Verification items for the finished model (mm, model axes). A direction names the side the tool comes from. Round coordinates to 2 decimals unless told otherwise and drop trailing zeros. Order: outer loops, then holes, each group sorted by start corner. A loop starts at its lowest first (then second) coordinate and runs counter-clockwise, first axis right, second up. Notation, with made-up numbers: (34.25, 31) -> (47.25, 31) arc R5 ccw to (47.25, 36) -> close; hole circle Ø4 at (31, 1). An arc over 180 degrees is marked (long way). Put each result on its own line as item: value.
```python
from build123d import *

# Parameters (mm, degrees)
F1_DEPTH       = 27.5
F0_R           = 8
F2_DEPTH       = 9.5
F5_D           = 3
F5_CSINK_D     = 8
F5_CSINK_ANGLE = 90
F6_W           = 26
F6_H           = 50
F6_R           = 1.5
F7_DEPTH       = 5


with BuildPart() as f1:
    # F0 (on Front) → F1 (new body, symmetric)
    with BuildSketch(Plane.XZ):
        Polygon((-15, 4.5), (-15, -4.5), (15, -4.5), (15, 0.0487750938), (15, 4.5), align=None)
    extrude(amount=F1_DEPTH, both=True)

    # F0 (on Front) → F2 (join, symmetric)
    with BuildSketch(Plane.XZ):
        with BuildLine():
            Line((15, 4.5), (15, 0.0487750938))
            Line((15, 0.0487750938), (26.0270317086, 0.0487750938))
            ThreePointArc((26.0270317086, 0.0487750938), (20.4485510909, 1.7874477446), (16.5475113082, 6.1376566135))
            ThreePointArc((16.5475113082, 6.1376566135), (16.1265778305, 4.9854273341), (15, 4.5))
        make_face()
        with BuildLine():
            ThreePointArc((16.5475113082, 6.1376566135), (20.4485510909, 1.7874477446), (26.0270317086, 0.0487750938))
            ThreePointArc((26.0270317086, 0.0487750938), (34.040923726, 3.1360416589), (37.393363731, 11.0426734401))
            ThreePointArc((37.393363731, 11.0426734401), (24.4033695136, 21.8611725511), (16.1133777283, 7.1283551362))
            ThreePointArc((16.1133777283, 7.1283551362), (16.4196666887, 6.6721038843), (16.5475113082, 6.1376566135))
        make_face()
        with Locations((26.393363731, 11.0426734401)):
            Circle(F0_R, mode=Mode.SUBTRACT)
    extrude(amount=F2_DEPTH, both=True)

    # F5 (through all)
    with Locations(Plane.XY.offset(4.5)):
        with Locations((3, 18.5), (3, -18.5)):
            CounterSinkHole(F5_D / 2, F5_CSINK_D / 2, counter_sink_angle=F5_CSINK_ANGLE)

    # F6 (on face) → F7 (cut)
    with BuildSketch(Plane(origin=(0, 0, -4.5), x_dir=(1, 0, 0), z_dir=(0, 0, -1))):
        Rectangle(F6_W, F6_H)
        with Locations((3, -18.5)):
            Circle(F6_R, mode=Mode.SUBTRACT)
        with Locations((3, 18.5)):
            Circle(F6_R, mode=Mode.SUBTRACT)
    extrude(amount=-F7_DEPTH, mode=Mode.SUBTRACT)


solid = f1.part
```
Item 1: Release check for a two-part mould opening along Z. For faces 1 (the face through (0, 0, 0.5)), 2 (the face through (3, -17, 1)), 3 (the face through (3.35, -20.08, 2.12)), 4 (the face through (18.4, 0.1, 11.4)) record: pulls with the +Z half, pulls with the -Z half, needs draft (parallel to the pull), parting line crosses it, or undercut.
Geometry check:
face 1: pulls with the -Z half
face 2: needs draft
face 3: pulls with the +Z half
face 4: undercut
Item 2: Material ranges on line 1 along Y through (x, z) = (3, 1.6); line 2 along X through (y, z) = (18.5, 1.3); line 3 along Y through (x, z) = (3, 0), recorded low to high.
Geometry check:
line 1: -27.5 to -20, -17 to 17, 20 to 27.5
line 2: -15 to 1.5, 4.5 to 15
line 3: -27.5 to -25, 25 to 27.5
Item 3: Depth check by flat-ended pin: pin 1 Ø1.5 at (y, z) = (9, -1) entering from +X; pin 2 Ø1.5 at (y, z) = (-7, 5.5) entering from +X; pin 3 Ø4 at (x, y) = (3, -18.5) entering from -Z; pin 4 Ø13 at (x, z) = (26.39, 11.04) entering from +Y. Enter the tip coordinate at first touch or a pass-through.
Geometry check:
pin 1: x = 15
pin 2: x = 36.29
pin 3: z = 0.5
pin 4: through
Item 4: Tool access check on faces 5 (the face through (0, 0, 4.5)), 6 (the face through (0, -25, -2)), 7 (the face through (20, 0, 0.049)), 8 (the face through (18.6, -9.5, 13.6)), 9 (the face through (18.6, 9.5, 13.6)). Record the directions out of +Z, -Z, +X, -X, +Y, -Y that give a thin tool (end or side, any length) a straight path to the whole face; none if there is none.
Geometry check:
face 5: +Z, -X, +Y, -Y
face 6: -Z
face 7: -Z, +X, +Y, -Y
face 8: +Z, -Z, +X, -Y
face 9: +Z, -Z, +X, +Y
Item 5: Sectioned sample at A-A, the plane y = 18.5. Record the boundary of the cut face in (x, z).
Geometry check:
outline: (-15, -4.5) -> (-13, -4.5) -> (-13, 0.5) -> (1.5, 0.5) -> (1.5, 2) -> (-1, 4.5) -> (-15, 4.5) -> close; (4.5, 0.5) -> (13, 0.5) -> (13, -4.5) -> (15, -4.5) -> (15, 4.5) -> (7, 4.5) -> (4.5, 2) -> close
Item 6: Sectioned sample at B-B, the plane x = 3. Record the boundary of the cut face in (y, z).
Geometry check:
outline: (-27.5, -4.5) -> (-25, -4.5) -> (-25, 0.5) -> (-20, 0.5) -> (-20, 2) -> (-22.5, 4.5) -> (-27.5, 4.5) -> close; (-17, 0.5) -> (17, 0.5) -> (17, 2) -> (14.5, 4.5) -> (-14.5, 4.5) -> (-17, 2) -> close; (20, 0.5) -> (25, 0.5) -> (25, -4.5) -> (27.5, -4.5) -> (27.5, 4.5) -> (22.5, 4.5) -> (20, 2) -> close
Item 7: Sectioned sample at D-D, the plane z = 16.5. Record the boundary of the cut face in (x, y), then the cut area to 3 significant figures.
Geometry check:
outline: (16.84, -9.5) -> (20.54, -9.5) -> (20.54, 9.5) -> (16.84, 9.5) -> close; (32.24, -9.5) -> (35.94, -9.5) -> (35.94, 9.5) -> (32.24, 9.5) -> close
area: 141 mm2
Item 8: Sectioned sample at C-C, the plane x = 29. Record the boundary of the cut face in (y, z).
Geometry check:
outline: (-9.5, 0.36) -> (9.5, 0.36) -> (9.5, 3.48) -> (-9.5, 3.48) -> close; (-9.5, 18.61) -> (9.5, 18.61) -> (9.5, 21.73) -> (-9.5, 21.73) -> close
